Source: three-view drawing plus pictorial views. Frame: mm from the lowest corner of the part. A direction names the side the tool comes from. Give positions to 0.01 mm unless a question says otherwise; leave off trailing zeros. Order: outer loops, then holes, each group sorted by start corner. A loop starts at its lowest first (then second) coordinate and runs counter-clockwise, first axis right, second up. Notation, with made-up numbers: (5, 50.5) - (43, 50.5) arc R10 ccw to (43, 68.5) - close; hole circle Ø11 at (8.25, 17.5). An arc over 180 degrees is marked (long way). Answer in a Markdown table with one row per item. Add a question column.
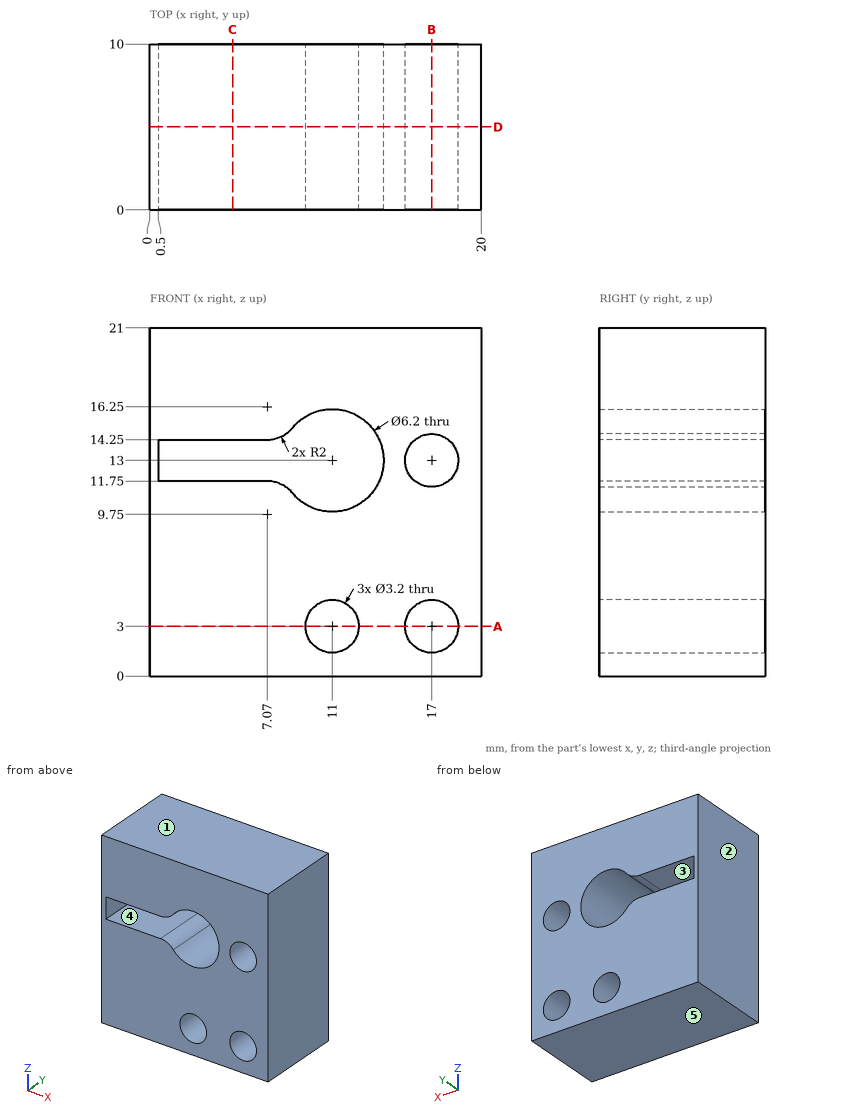
Q1. Section B-B, the plane x = 17. Return loops of the section in (y, z), then the cut area to 3 significant figures.
Q2. Section C-C, the plane x = 5. Return loops of the section in (y, z), then the cut area to 3 significant figures.
Q3. Pull-direction query (Z, two-part tool) for the marked faces 1, 2 and 3; classes: +Z half, -Z half, draft (parallel to the pull), parting line (faces both ways), or undercut.
Q4. Section D-D, the plane y = 5. State how many separate pieces and enclosed holes the cut face has, then the cut area to 3 significant figures.
Q5. Section A-A, the plane z = 3. Return loops of the section in (x, y), then the cut area to 3 significant figures.
Q6. Line query: probe 1 along X at (y, z) = (3, 2); probe 2 along Z at (x, y) = (18, 3); probe 3 along X at (y, z) = (3.25, 3.75). Output: solid intervals per line, ascending.
Q7. Contact query for a flat-ended pin moving along its axis: P1, Ø2.5, axis at x = 17, z = 3, coming from the -Y side. Output: stop coordinate, or through.
Q8. Access query for the marked faces 4 and 5. Directions: +Z, -Z, +X, -X, +Y, -Y. A direction counts if a zero-diameter tool reaches every point of the face in a straight line with its end or side. Return the directions, or none.
Computed:
| question | item | result |
|---|---|---|
| 1 | outline | (0, 0) - (10, 0) - (10, 1.4) - (0, 1.4) - close; (0, 4.6) - (10, 4.6) - (10, 11.4) - (0, 11.4) - close; (0, 14.6) - (10, 14.6) - (10, 21) - (0, 21) - close |
| 1 | area | 146 mm^2 |
| 2 | outline | (0, 0) - (10, 0) - (10, 11.75) - (0, 11.75) - close; (0, 14.25) - (10, 14.25) - (10, 21) - (0, 21) - close |
| 2 | area | 185 mm^2 |
| 3 | face 1 | +Z half |
| 3 | face 2 | draft |
| 3 | face 3 | undercut |
| 4 | separate pieces | 1 |
| 4 | enclosed holes | 4 |
| 4 | area | 347 mm^2 |
| 5 | outline | (0, 0) - (9.4, 0) - (9.4, 10) - (0, 10) - close; (12.6, 0) - (15.4, 0) - (15.4, 10) - (12.6, 10) - close; (18.6, 0) - (20, 0) - (20, 10) - (18.6, 10) - close |
| 5 | area | 136 mm^2 |
| 6 | probe 1 | x = 0 to 9.75, 12.25 to 15.75, 18.25 to 20 |
| 6 | probe 2 | z = 0 to 1.75, 4.25 to 11.75, 14.25 to 21 |
| 6 | probe 3 | x = 0 to 9.59, 12.41 to 15.59, 18.41 to 20 |
| 7 | P1 | passes through |
| 8 | face 4 | +Y, -Y |
| 8 | face 5 | -Z, +X, -X, +Y, -Y |
